```python
from build123d import *

# Parameters (mm, degrees)
F0_W     = 1400
F0_H     = 800
F1_DEPTH = 25
F2_SIZE2 = 12.5
F2_SIZE  = 40


with BuildPart() as f1:
    # F0 (on Top) → F1 (new body)
    with BuildSketch(Plane.XY):
        with Locations((-700, 400)):
            Rectangle(F0_W, F0_H)
    extrude(amount=F1_DEPTH)

    # F2
    f2_edges = [f1.edges().sort_by_distance(p)[0] for p in [
        (-700, 0, 0),
        (0, 400, 0),
        (-700, 800, 0),
        (-1400, 400, 0),
    ]]
    f2_side = f1.faces().sort_by_distance((-700, 400, 0))[0]
    chamfer(f2_edges, length=F2_SIZE, length2=F2_SIZE2, reference=f2_side)


solid = f1.part
```
Model file for the job. Use its own axes, mm. Give positions to 0.01 mm unless a question says otherwise; leave off trailing zeros. Loops run counter-clockwise (first coordinate to the right, second up) from the corner with the lowest first, then second, coordinate; pieces in that order, holes last. Notation, with made-up numbers: (74.25, 3) - (131.25, 3) arc R34 cw to (131.25, 40) - close; hole circle Ø11 at (76.5, -20.75). An arc over 180 degrees is marked (long way). One line per item, written item: value. Start each with the question number.
1. Slice it at A-A (x = -1137). List the corners of the cut face in (y, z).
2. Pull direction Z, two halves, no side cores. Call faces 1 (the flat face through (-710, 406, 25)), 2 (the flat face through (-709, 405, 0)): pulls with the +Z half, pulls with the -Z half, needs draft (parallel to the pull), parting line crosses it, or undercut.
3. Slice it at B-B (z = 6.75). List the corners of the cut face in (x, y), plus the area to 3 significant figures.
Solution:
1. outline: (0, 12.5) - (40, 0) - (760, 0) - (800, 12.5) - (800, 25) - (0, 25) - close
2. face 1: pulls with the +Z half
2. face 2: pulls with the -Z half
3. outline: (-1381.6, 18.4) - (-18.4, 18.4) - (-18.4, 781.6) - (-1381.6, 781.6) - close
3. area: 1,040,000 mm^2
